For this review, take the finished solid that the model builds, in its own axes (mm). Give positions to 0.01 mm unless a question says otherwise; leave off trailing zeros. Loops run counter-clockwise (first coordinate to the right, second up) from the corner with the lowest first, then second, coordinate; pieces in that order, holes last. Notation, with made-up numbers: M 16,9.25 L 58,9.25 A18 cw 58,33.25 Z; hole C 78.5,83 d11. An arc over 180 degrees is marked long. Use CSV: the item, a comma, the result in double quotes. Start each with the question number.
1. Take a section at D-D, the plane x = 10.75. Write out the cut boundary in (y, z) (3 decimals).
2. Take a section at C-C, the plane z = -3.25. Write out the cut boundary in (x, y), and give its area (3 significant figures).
3. Insertion check: P1, Ø1.8, axis at y = 9.525, z = -16.129, coming from the +X side; P2, Ø3, axis at y = 10, z = -16, coming from the -X side; P3, Ø1, axis at y = 6.5, z = -8, coming from the +X side. Each pin has a flat end and moves straight along its axis. Give the tip position at first contact, or say it passes through.
4. Take a section at A-A, the plane x = 12. Write out the cut boundary in (y, z) (3 decimals), and give its area (3 significant figures).
5. To check wall thickness, follow line 1 (Z direction, x = 10, y = 3.25); line 2 (Y direction, x = 10.5, z = -16.25); line 3 (Z direction, x = 10.5, y = 3.75). State the ranges of each line that lie inside material, in increasing order. Write a range as [from, to].
6. The part is to be moulded in two halves that separate along Z. For faces 1 (the face through (9.57, 3.63, -17.56)), 2 (the face through (9.569, 11.012, -2.98)), 3 (the face through (12.7, 6, -3)), 4 (the face through (9, 6, -19.05)), say which applies: pulls with the +Z half, pulls with the -Z half, needs draft (parallel to the pull), parting line crosses it, or undercut.
7. Take a section at B-B, the plane y = 3.5. Write out the cut boundary in (x, z) (3 decimals).
from build123d import *

# Parameters (mm, degrees)
SKETCH1_W           = 12.7
SKETCH1_H           = 19.05
BOSS_EXTRUDE1_DEPTH = 12.7
CUT_EXTRUDE2_DEPTH  = 12.7
SKETCH5_R           = 1.5
CUT_EXTRUDE3_DEPTH  = 12.7
CUT_EXTRUDE4_DEPTH  = 12.7
SKETCH7_W           = 12.213119959
SKETCH7_H           = 9.608468088
CUT_EXTRUDE5_DEPTH  = 12.7


with BuildPart() as part:
    # Sketch1 → Boss-Extrude1 (new body)
    with BuildSketch(Plane(origin=(0, 0, 0), x_dir=(1, 0, 0), z_dir=(0, 1, 0))):
        with Locations((6.35, 9.525)):
            Rectangle(SKETCH1_W, SKETCH1_H)
    extrude(amount=BOSS_EXTRUDE1_DEPTH)

    # Sketch4 → Cut-Extrude2 (cut)
    with BuildSketch(Plane(origin=(0, 12.7, 0), x_dir=(1, 0, 0), z_dir=(0, 1, 0))):
        Polygon((0, 19.05), (0, 9.525), (6.35, 19.05), align=None)
        Polygon((6.35, 0), (0, 9.525), (0, 0), align=None)
        with BuildLine():
            Line((12.7, 5.932897552), (12.7, 13.117102448))
            ThreePointArc((12.7, 13.117102448), (10.16, 9.525), (12.7, 5.932897552))
        make_face()
        with BuildLine():
            ThreePointArc((17.78, 9.525), (16.169704526, 12.635851973), (12.7, 13.117102448))
            Line((12.7, 13.117102448), (12.7, 5.932897552))
            ThreePointArc((12.7, 5.932897552), (16.169704526, 6.414148027), (17.78, 9.525))
        make_face()
    extrude(amount=-CUT_EXTRUDE2_DEPTH, mode=Mode.SUBTRACT)

    # Sketch5 → Cut-Extrude3 (cut)
    with BuildSketch(Plane(origin=(12.7, 0, 0), x_dir=(0, 0, -1), z_dir=(1, 0, 0))):
        with Locations((3.175, 9.525)):
            Circle(SKETCH5_R)
        with Locations((16.129, 9.525)):
            Circle(SKETCH5_R)
        with Locations((16.129, 3.175)):
            Circle(SKETCH5_R)
        with Locations((3.175, 3.175)):
            Circle(SKETCH5_R)
    extrude(amount=-CUT_EXTRUDE3_DEPTH, mode=Mode.SUBTRACT)

    # Sketch6 → Cut-Extrude4 (cut)
    with BuildSketch(Plane.XZ):
        Polygon((6.35, 0), (6.35, -5.570300529), (2.636466314, -5.570300529), align=None)
    cut_extrude4 = extrude(amount=-CUT_EXTRUDE4_DEPTH, mode=Mode.SUBTRACT)

    # Mirror1: Cut-Extrude4 across plane
    add(cut_extrude4.mirror(Plane(origin=(0, 0, -9.525), x_dir=(1, 0, 0), z_dir=(0, 0, -1))), mode=Mode.SUBTRACT)

    # Sketch7 → Cut-Extrude5 (cut)
    with BuildSketch(Plane.XZ):
        with Locations((0.243440021, -8.675465427)):
            Rectangle(SKETCH7_W, SKETCH7_H)
    extrude(amount=-CUT_EXTRUDE5_DEPTH, mode=Mode.SUBTRACT)


solid = part.part
Result set:
1,outline,"M 0,-19.05 L 12.7,-19.05 L 12.7,-11.562 L 0,-11.562 Z; M 0,-7.488 L 12.7,-7.488 L 12.7,0 L 0,0 Z; hole C 3.175,-16.129 d3; hole C 3.175,-3.175 d3; hole C 9.525,-16.129 d3; hole C 9.525,-3.175 d3"
2,outline,"M 6.35,0 L 12.7,0 L 12.7,1.68 L 6.35,1.68 Z; M 6.35,4.67 L 12.7,4.67 L 12.7,8.03 L 6.35,8.03 Z; M 6.35,11.02 L 12.7,11.02 L 12.7,12.7 L 6.35,12.7 Z"
2,area,"42.6 mm2"
3,P1,"through"
3,P2,"x = 6.35"
3,P3,"x = 10.74"
4,outline,"M 0,-19.05 L 12.7,-19.05 L 12.7,-12.786 L 0,-12.786 Z; M 0,-6.264 L 12.7,-6.264 L 12.7,0 L 0,0 Z; hole C 3.175,-16.129 d3; hole C 3.175,-3.175 d3; hole C 9.525,-16.129 d3; hole C 9.525,-3.175 d3"
4,area,"131 mm2"
5,line 1,"[-19.05, -17.63], [-14.63, -4.67], [-1.68, 0]"
5,line 2,"[0, 1.68], [4.67, 8.03], [11.02, 12.7]"
5,line 3,"[-19.05, -17.51], [-14.74, -11.1], [-7.95, -4.56], [-1.79, 0]"
6,face 1,"undercut"
6,face 2,"undercut"
6,face 3,"needs draft"
6,face 4,"pulls with the -Z half"
7,outline,"M 6.35,-19.05 L 12.7,-19.05 L 12.7,-17.593 L 6.35,-17.593 Z; M 6.35,-14.665 L 12.7,-14.665 L 12.7,-13.117 A3.81 cw 12.7,-5.933 L 12.7,-4.639 L 6.35,-4.639 Z; M 6.35,-1.711 L 12.7,-1.711 L 12.7,0 L 6.35,0 Z"
